Part model, mm, in its own coordinate system. A direction names the side the tool comes from. Give positions to 0.01 mm unless a question says otherwise; leave off trailing zeros. Write each loop counter-clockwise with the first axis right and the second up, starting at its lowest first coordinate (ties: lowest second). Pieces come first, ordered by that corner, then holes. Notation, with made-up numbers: M 8.5,36.25 L 23.5,36.25 A8 ccw 23.5,41.25 Z; hole C 47.5,89.5 d9. An arc over 180 degrees is marked long. Use a Markdown table: item, result.
```python
from build123d import *

# Parameters (mm, degrees)
EXTRUDE2_DEPTH     = 1.537890625
SKETCH3_R          = 6.1515625
EXTRUDE1_DEPTH     = 0.85725
EXTRUDE1_DRAFT     = -5
SKETCH15_R         = 6.076562843
EXTRUDE3_DEPTH     = 4.85775
EXTRUDE3_TAPER     = 21.960198558
FILLET3_R          = 0.254
SKETCH4_R          = 3.175
CUT_EXTRUDE1_DEPTH = 23.225885864
CHAMFER1_SIZE      = 0.32146875
CHAMFER1_SIZE2     = 0.296735699
FILLET4_R          = 0.512630208


with BuildPart() as part:
    # Sketch13 → Extrude2 (new, symmetric)
    with BuildSketch(Plane(origin=(0, 0, 0), x_dir=(1, 0, 0), z_dir=(0, 1, 0))):
        with BuildLine():
            Line((3.773545526, 0.428625), (6.1515625, 0.428625))
            ThreePointArc((6.1515625, 0.428625), (8.590910612, 0.981496101), (10.553521716, 2.53205836))
            ThreePointArc((10.553521716, 2.53205836), (13.326559198, 7.495965423), (14.2875, 13.10013378))
            ThreePointArc((14.2875, 13.10013378), (14.187492334, 13.501242622), (13.91088161, 13.808449953))
            ThreePointArc((13.91088161, 13.808449953), (10.685615281, 15.346823078), (7.151500977, 15.875))
            ThreePointArc((7.151500977, 15.875), (6.631385147, 15.698444466), (6.326229714, 15.241747088))
            Line((6.326229714, 15.241747088), (3.773545526, 5.715))
            Line((3.773545526, 5.715), (3.773545526, 0.428625))
        make_face()
    extrude(amount=EXTRUDE2_DEPTH, both=True)

    # Fillet4
    fillet4_edges = [part.edges().sort_by_distance(p)[0] for p in [
        (8.590910612, 1.537890625, -0.981496101),
        (4.962554013, -1.537890625, -0.428625),
        (13.326559198, 1.537890625, -7.495965423),
        (14.187492334, 1.537890625, -13.501242622),
        (10.685615281, 1.537890625, -15.346823078),
        (6.631385147, 1.537890625, -15.698444466),
        (5.04988762, 1.537890625, -10.478373544),
        (4.962554013, 1.537890625, -0.428625),
        (5.04988762, -1.537890625, -10.478373544),
        (6.631385147, -1.537890625, -15.698444466),
        (10.685615281, -1.537890625, -15.346823078),
        (14.187492334, -1.537890625, -13.501242622),
        (13.326559198, -1.537890625, -7.495965423),
        (8.590910612, -1.537890625, -0.981496101),
    ]]
    fillet(fillet4_edges, radius=FILLET4_R)


with BuildPart() as body_2:
    # Sketch3 → Extrude1 (with draft: the straight prism first)
    with BuildSketch(Plane.XY):
        Circle(SKETCH3_R)
    extrude(amount=-EXTRUDE1_DEPTH)
    # Extrude1: the draft: its side faces are tilted about the plane it starts from
    extrude1_sides = [body_2.faces().sort_by_distance(p)[0] for p in [
        (-6.1515625, 0, -0.428625),
    ]]
    draft(extrude1_sides, Plane.XY, EXTRUDE1_DRAFT)

    # Sketch15 → Extrude3 (add)
    with BuildSketch(Plane(origin=(0, 0, -0.85725), x_dir=(-1, 0, 0), z_dir=(0, 0, -1))):
        Circle(SKETCH15_R)
    extrude(amount=EXTRUDE3_DEPTH, taper=EXTRUDE3_TAPER)

    # Fillet3
    fillet3_edges = [body_2.edges().sort_by_distance(p)[0] for p in [
        (4.117828705, 0, -5.715),
    ]]
    fillet(fillet3_edges, radius=FILLET3_R)

    # Sketch4 → Cut-Extrude1 (cut, through all)
    with BuildSketch(Plane.XY):
        Circle(SKETCH4_R)
    extrude(amount=-CUT_EXTRUDE1_DEPTH, mode=Mode.SUBTRACT)

    # Chamfer1
    chamfer1_edges = [body_2.edges().sort_by_distance(p)[0] for p in [
        (-6.1515625, 0, 0),
    ]]
    chamfer1_side = [body_2.faces().sort_by_distance(p)[0] for p in [
        (-6.114062672, 0, -0.428625),
    ]]
    chamfer(chamfer1_edges, length=CHAMFER1_SIZE, length2=CHAMFER1_SIZE2, reference=chamfer1_side[0])


with BuildPart() as body_3:
    # Mirror6: mirrored copy
    add(part.part.mirror(Plane(origin=(0, 0, 0), x_dir=(0, 0, 1), z_dir=(1, 0, 0))))

    # Combine2: union part, body 2
    add(part.part)
    add(body_2.part)


solid = body_3.part
```
1. Drop flat-ended pins along their axis: P1, Ø7.5, axis at x = 9.5, z = -11, coming from the -Y side; P2, Ø5, axis at x = -9.5, z = -10, coming from the +Y side; P3, Ø4, axis at y = -4.5, z = -3, coming from the +X side. Give the stop position or say it passes through.
Findings below:
| item | result |
|---|---|
| P1 | y = -1.54 |
| P2 | y = 1.54 |
| P3 | x = 4.9 |
2. Two-plate mould, pull along Y, no slides. Class faces 4 (the cylindrical face through (-5.105, 1.392, -10.088)), 5 (the cylindrical face through (-0.69, -3.1, -2.82)), 6 (the cylindrical face through (-10.734, 0.014, -15.332)), 7 (the cylindrical face through (-5.097, -1.384, -10.09)): released by +Y, released by -Y, zero draft, split by the parting line, or undercut.
Findings below:
| item | result |
|---|---|
| face 4 | released by +Y |
| face 5 | undercut |
| face 6 | zero draft |
| face 7 | released by -Y |
3. Cut at A-A, the plane x = 0. Give the cut face in (y, z) (3 decimals), then the cut area to 3 significant figures.
Findings below:
| item | result |
|---|---|
| outline | M -6.124,-0.32 L -6.077,-0.857 L -4.182,-5.556 A0.254 ccw -3.946,-5.715 L -3.175,-5.715 L -3.175,0 L -5.855,0 Z; M 3.175,-5.715 L 3.946,-5.715 A0.254 ccw 4.182,-5.556 L 6.077,-0.857 L 6.124,-0.32 L 5.855,0 L 3.175,0 Z |
| area | 23.6 mm2 |
4. Drill centre lines: L1, parallel to Y at x = -6.25, z = -8.25; L2, parallel to X at y = -0.5, z = -14.75; L3, parallel to X at y = 0.25, z = -5.5. Where is each one in solid material? Low to high.
Findings below:
| item | result |
|---|---|
| L1 | -1.54 to 1.54 |
| L2 | -12.24 to -6.19, 6.19 to 12.24 |
| L3 | -12.47 to -3.17, 3.17 to 12.47 |
5. Tool access for faces 1 (the cylindrical face through (5.105, 1.392, -10.088)), 2 (the cylindrical face through (-6.638, 0.014, -15.703)), 3 (the flat face through (9, -1.538, -8)): list every direction of +Z, -Z, +X, -X, +Y, -Y with a clear straight run to the whole face (end or side of a thin tool).
Findings below:
| item | result |
|---|---|
| face 1 | -Z, +Y |
| face 2 | -Z, +Y, -Y |
| face 3 | -Z, +X, -Y |
